For this review, take the finished solid that the model builds, in its own axes (mm). A direction names the side the tool comes from. Give positions to 0.01 mm unless a question says otherwise; leave off trailing zeros. Write each loop counter-clockwise with the first axis right and the second up, starting at its lowest first coordinate (ties: lowest second). Pieces come first, ordered by that corner, then holes.
from build123d import *

# Parameters (mm, degrees)
SKETCH1_W               = 40.8
SKETCH1_H               = 40.8
SKETCH1_W_2             = 38.4
SKETCH1_H_2             = 38.4
BOSS_EXTRUDE1_DEPTH     = 1.7
SKETCH2_W               = 40.8
SKETCH2_H               = 40.8
SKETCH2_R               = 2.35
BOSS_EXTRUDE2_DEPTH     = 3.8
SKETCH3_W               = 40.8
SKETCH3_H               = 40.8
BOSS_EXTRUDE3_DEPTH     = 1.2
SKETCH4_W               = 23
SKETCH4_H               = 10
CUT_EXTRUDE1_DEPTH      = 30.617731176
CUT_EXTRUDE2_DEPTH      = 30.369542046
CUT_EXTRUDE2_DEPTH_BACK = 30.369542046
SKETCH6_R               = 1.525
CUT_EXTRUDE3_DEPTH      = 30.280027322
FILLET1_R               = 0.4


with BuildPart() as part:
    # Sketch1 → Boss-Extrude1 (new body)
    with BuildSketch(Plane.XY):
        Rectangle(SKETCH1_W, SKETCH1_H)
        Rectangle(SKETCH1_W_2, SKETCH1_H_2, mode=Mode.SUBTRACT)
    extrude(amount=BOSS_EXTRUDE1_DEPTH)

    # Sketch2 → Boss-Extrude2 (add)
    # profile 1 of 9: a face of its own
    with BuildSketch(Plane(origin=(0, 0, 0), x_dir=(-1, 0, 0), z_dir=(0, 0, -1))):
        Rectangle(SKETCH2_W, SKETCH2_H)
        Polygon((-19.2, -15.876598128), (-19.2, 15.876598128), (-19.2, 19.2), (-15.876598128, 19.2), (15.876598128, 19.2), (19.2, 19.2), (19.2, 15.876598128), (19.2, -15.876598128), (19.2, -19.2), (15.876598128, -19.2), (-15.876598128, -19.2), (-19.2, -19.2), align=None, mode=Mode.SUBTRACT)
    # profile 2 of 9: a face of its own
    with BuildSketch(Plane(origin=(0, 0, 0), x_dir=(-1, 0, 0), z_dir=(0, 0, -1))):
        with BuildLine():
            Line((-19.2, 15.876598128), (-16.661700936, 13.338299064))
            ThreePointArc((-16.661700936, 13.338299064), (-16.661700936, 16.661700936), (-13.338299064, 16.661700936))
            Line((-13.338299064, 16.661700936), (-15.876598128, 19.2))
            Line((-15.876598128, 19.2), (-19.2, 19.2))
            Line((-19.2, 19.2), (-19.2, 15.876598128))
        make_face()
    # profile 3 of 9: a face of its own
    with BuildSketch(Plane(origin=(0, 0, 0), x_dir=(-1, 0, 0), z_dir=(0, 0, -1))):
        with BuildLine():
            Line((19.2, 19.2), (15.876598128, 19.2))
            Line((15.876598128, 19.2), (13.338299064, 16.661700936))
            ThreePointArc((13.338299064, 16.661700936), (15.899306066, 17.171116901), (17.35, 15))
            ThreePointArc((17.35, 15), (17.171116901, 14.100693934), (16.661700936, 13.338299064))
            Line((16.661700936, 13.338299064), (19.2, 15.876598128))
            Line((19.2, 15.876598128), (19.2, 19.2))
        make_face()
    # profile 4 of 9: a face of its own
    with BuildSketch(Plane(origin=(0, 0, 0), x_dir=(-1, 0, 0), z_dir=(0, 0, -1))):
        with Locations((15, 15)):
            Circle(SKETCH2_R)
    # profile 5 of 9: a face of its own
    with BuildSketch(Plane(origin=(0, 0, 0), x_dir=(-1, 0, 0), z_dir=(0, 0, -1))):
        with Locations((-15, 15)):
            Circle(SKETCH2_R)
    # profile 6 of 9: a face of its own
    with BuildSketch(Plane(origin=(0, 0, 0), x_dir=(-1, 0, 0), z_dir=(0, 0, -1))):
        with Locations((15, -15)):
            Circle(SKETCH2_R)
    # profile 7 of 9: a face of its own
    with BuildSketch(Plane(origin=(0, 0, 0), x_dir=(-1, 0, 0), z_dir=(0, 0, -1))):
        with BuildLine():
            Line((13.338299064, -16.661700936), (15.876598128, -19.2))
            Line((15.876598128, -19.2), (19.2, -19.2))
            Line((19.2, -19.2), (19.2, -15.876598128))
            Line((19.2, -15.876598128), (16.661700936, -13.338299064))
            ThreePointArc((16.661700936, -13.338299064), (17.171116901, -14.100693934), (17.35, -15))
            ThreePointArc((17.35, -15), (15.899306066, -17.171116901), (13.338299064, -16.661700936))
        make_face()
    # profile 8 of 9: a face of its own
    with BuildSketch(Plane(origin=(0, 0, 0), x_dir=(-1, 0, 0), z_dir=(0, 0, -1))):
        with Locations((-15, -15)):
            Circle(SKETCH2_R)
    # profile 9 of 9: a face of its own
    with BuildSketch(Plane(origin=(0, 0, 0), x_dir=(-1, 0, 0), z_dir=(0, 0, -1))):
        with BuildLine():
            Line((-16.661700936, -13.338299064), (-19.2, -15.876598128))
            Line((-19.2, -15.876598128), (-19.2, -19.2))
            Line((-19.2, -19.2), (-15.876598128, -19.2))
            Line((-15.876598128, -19.2), (-13.338299064, -16.661700936))
            ThreePointArc((-13.338299064, -16.661700936), (-16.661700936, -16.661700936), (-16.661700936, -13.338299064))
        make_face()
    extrude(amount=BOSS_EXTRUDE2_DEPTH)

    # Sketch3 → Boss-Extrude3 (add)
    with BuildSketch(Plane(origin=(0, 0, -3.8), x_dir=(-1, 0, 0), z_dir=(0, 0, -1))):
        Rectangle(SKETCH3_W, SKETCH3_H)
    extrude(amount=BOSS_EXTRUDE3_DEPTH)

    # Sketch4 → Cut-Extrude1 (cut, through all)
    with BuildSketch(Plane(origin=(0, 0, -5), x_dir=(-1, 0, 0), z_dir=(0, 0, -1))):
        with Locations((0, -20.4)):
            Rectangle(SKETCH4_W, SKETCH4_H)
    extrude(amount=-CUT_EXTRUDE1_DEPTH, mode=Mode.SUBTRACT)

    # Sketch5 → Cut-Extrude2 (cut, two sides: drawn at the far end of the back side and taken through both)
    with BuildSketch(Plane.XY.offset(-3.8).offset(-CUT_EXTRUDE2_DEPTH_BACK)):
        Polygon((-11.5, -15.4), (-17.658402739, -21.558402739), (17.658402739, -21.558402739), (11.5, -15.4), align=None)
    extrude(amount=CUT_EXTRUDE2_DEPTH + CUT_EXTRUDE2_DEPTH_BACK, mode=Mode.SUBTRACT)

    # Sketch6 → Cut-Extrude3 (cut, through all)
    with BuildSketch(Plane.XY):
        with Locations((-15, -15)):
            Circle(SKETCH6_R)
        with Locations((-15, 15)):
            Circle(SKETCH6_R)
        with Locations((15, 15)):
            Circle(SKETCH6_R)
        with Locations((15, -15)):
            Circle(SKETCH6_R)
    extrude(amount=-CUT_EXTRUDE3_DEPTH, mode=Mode.SUBTRACT)

    # Fillet1
    fillet1_edges = [part.edges().sort_by_distance(p)[0] for p in [
        (-14.607448596, 17.930850468, 0),
        (-17.930850468, -14.607448596, 0),
        (14.607448596, -17.930850468, 0),
        (17.930850468, 14.607448596, 0),
        (17.930850468, -14.607448596, 0),
        (13.338299064, 13.338299064, 0),
        (14.607448596, 17.930850468, 0),
        (-13.338299064, 13.338299064, 0),
        (-17.930850468, 14.607448596, 0),
        (-13.338299064, -13.338299064, 0),
        (-14.607448596, -17.930850468, 0),
        (13.338299064, -13.338299064, 0),
    ]]
    fillet(fillet1_edges, radius=FILLET1_R)


solid = part.part
(1) We need section A-A (z = -3). Write out the cut boundary in (x, y) (3 decimals).
(2) Clearance check with flat-ended pins moving along their axes: pin 1 Ø4 at (x, y) = (15, 15) entering from +Z; pin 2 Ø1.8 at (x, y) = (-15, -15) entering from -Z; pin 3 Ø1 at (x, z) = (5, -4) entering from -Y. State where each tip first meets the part, or that it passes through.
(3) Tool access review of faces 4 (the cylindrical face through (-18.007, 14.854, -0.114)), 5 (the cylindrical face through (-14.296, 13.647, -2.465)), 6 (the flat face through (-15.6, -19.5, -3.2)): name each direction out of +Z, -Z, +X, -X, +Y, -Y from which nothing blocks a thin tool from reaching the whole face with its end or side.
(4) We need section B-B (y = 3.5). Write out the cut boundary in (x, z), and give its area (3 significant figures).
(5) We need section C-C (x = -5). Write out the cut boundary in (y, z), and give its area (3 significant figures).
(6) The part is to be moulded in two halves that separate along Y. For faces 1 (the flat face through (0, 0, -5)), 2 (the flat face through (0, 20.4, -2)), 3 (the flat face through (14.59, 17.913, -2.076)), say which applies: +Y half, -Y half, draft (parallel to the pull), parting line (faces both ways), or undercut.
(7) For L1, parallel to X at y = -5, z = -2.5; L2, parallel to Y at x = -15, z = -2 (3 decimals); L3, parallel to Y at x = -13, z = -1.25, list the stretches that pass through material, from the lowest coordinate up.
The answers:
1. outline: (-20.4, -20.4) - (-16.5, -20.4) - (-15.3, -19.2) - (-15.877, -19.2) - (-13.338, -16.662) arc R2.35 ccw to (-16.662, -13.338) - (-19.2, -15.877) - (-19.2, 15.877) - (-16.662, 13.338) arc R2.35 ccw to (-13.338, 16.662) - (-15.877, 19.2) - (15.877, 19.2) - (13.338, 16.662) arc R2.35 ccw to (16.662, 13.338) - (19.2, 15.877) - (19.2, -15.877) - (16.662, -13.338) arc R2.35 ccw to (13.338, -16.662) - (15.877, -19.2) - (15.3, -19.2) - (16.5, -20.4) - (20.4, -20.4) - (20.4, 20.4) - (-20.4, 20.4) - close; hole circle Ø3.05 at (-15, -15); hole circle Ø3.05 at (-15, 15); hole circle Ø3.05 at (15, -15); hole circle Ø3.05 at (15, 15)
2. pin 1: stops at z = 0
2. pin 2: passes through
2. pin 3: stops at y = -15.4
3. face 4: +Z
3. face 5: +Z, -Z
3. face 6: +Z, -Z, -Y
4. outline: (-20.4, -5) - (20.4, -5) - (20.4, 1.7) - (19.2, 1.7) - (19.2, -3.8) - (-19.2, -3.8) - (-19.2, 1.7) - (-20.4, 1.7) - close
4. area: 62.2 mm2
5. outline: (-15.4, -5) - (20.4, -5) - (20.4, 1.7) - (19.2, 1.7) - (19.2, -3.8) - (-15.4, -3.8) - close
5. area: 49.6 mm2
6. face 1: draft
6. face 2: +Y half
6. face 3: undercut
7. L1: x = -20.4 to -19.2, 19.2 to 20.4
7. L2: y = -18.323 to -16.525, -13.475 to -12.65, 12.65 to 13.475, 16.525 to 18.323, 19.2 to 20.4
7. L3: y = -16.23 to -13.77, 13.77 to 16.23, 19.2 to 20.4
